Work out the finished part from the listing and answer in its coordinate system (mm). A direction names the side the tool comes from. Give positions to 0.01 mm unless a question says otherwise; leave off trailing zeros. Loops run counter-clockwise (first coordinate to the right, second up) from the corner with the lowest first, then second, coordinate; pieces in that order, holes last. Notation, with made-up numbers: M -28,22.5 L 13,22.5 A15 ccw 13,30.5 Z; hole C 54,-29 d2. An arc over 180 degrees is marked long. Use a Markdown table: item, result.
```python
from build123d import *

# Parameters (mm, degrees)
SKETCH1_R           = 25
BOSS_EXTRUDE1_DEPTH = 12
BOSS_EXTRUDE2_START = 12
SKETCH2_R           = 14
BOSS_EXTRUDE2_DEPTH = 7
CUT_EXTRUDE1_START  = 19
SKETCH3_R           = 11.15
CUT_EXTRUDE1_DEPTH  = 2.1
FILLET1_R           = 10
FILLET2_R           = 4
SKETCH4_R           = 11
BOSS_EXTRUDE3_DEPTH = 8
CUT_EXTRUDE2_START  = 16.9
SKETCH5_R           = 2.05
CUT_EXTRUDE2_DEPTH  = 9
SKETCH6_R           = 2.05
CUT_EXTRUDE3_DEPTH  = 9


with BuildPart() as part:
    # Sketch1 → Boss-Extrude1 (new body)
    with BuildSketch(Plane.XY):
        Circle(SKETCH1_R)
    extrude(amount=BOSS_EXTRUDE1_DEPTH)

    # Sketch2 → Boss-Extrude2 (add)
    with BuildSketch(Plane.XY.offset(BOSS_EXTRUDE2_START)):
        Circle(SKETCH2_R)
    extrude(amount=BOSS_EXTRUDE2_DEPTH)

    # Sketch3 → Cut-Extrude1 (cut)
    with BuildSketch(Plane.XY.offset(CUT_EXTRUDE1_START)):
        Circle(SKETCH3_R)
    extrude(amount=-CUT_EXTRUDE1_DEPTH, mode=Mode.SUBTRACT)

    # Fillet1
    # the kernel refuses this fillet: 10 mm, written as the material it adds along each edge
    with BuildSketch(Plane(origin=(0, 0, 12), x_dir=(1, 0, 0), z_dir=(0, -1, 0))) as fillet1_piece_1:
        with BuildLine():
            CenterArc((23.539392014, 10), FILLET1_R, 197.457603124, 72.542396876)
            Line((14, 7), (13.80921216, 6.94))
            ThreePointArc((13.80921216, 6.94), (13.8, 3.5), (13.8, 0))
            Line((13.8, 0), (14, -0.2))
            Line((14, -0.2), (23.539392014, -0.2))
            Line((23.539392014, -0.2), (23.539392014, 0))
        make_face()
    revolve(axis=Axis((0, 0, 12), (0, 0, 1)))

    # Fillet2
    fillet2_edges = [part.edges().sort_by_distance(p)[0] for p in [
        (-25, 0, 12),
    ]]
    fillet(fillet2_edges, radius=FILLET2_R)

    # Sketch4 → Boss-Extrude3 (add)
    with BuildSketch(Plane.XY):
        Circle(SKETCH4_R)
    extrude(amount=-BOSS_EXTRUDE3_DEPTH)

    # Sketch5 → Cut-Extrude2 (cut)
    with BuildSketch(Plane.XY.offset(CUT_EXTRUDE2_START)):
        with Locations((0, 8)):
            Circle(SKETCH5_R)
        with Locations((8, 0)):
            Circle(SKETCH5_R)
        with Locations((0, -8)):
            Circle(SKETCH5_R)
        with Locations((-8, 0)):
            Circle(SKETCH5_R)
    extrude(amount=-CUT_EXTRUDE2_DEPTH, mode=Mode.SUBTRACT)

    # Sketch6 → Cut-Extrude3 (cut)
    with BuildSketch(Plane.XY):
        with Locations((0, 18)):
            Circle(SKETCH6_R)
        with Locations((18, 0)):
            Circle(SKETCH6_R)
        with Locations((0, -18)):
            Circle(SKETCH6_R)
        with Locations((-18, 0)):
            Circle(SKETCH6_R)
    extrude(amount=CUT_EXTRUDE3_DEPTH, mode=Mode.SUBTRACT)


solid = part.part
```
(1) A cutting plane is placed at A-A (z = 7.25). Write down the section's boundary in (x, y), and give its area (3 significant figures).
Entries:
| item | result |
|---|---|
| outline | C 0,0 d50; hole C -18,0 d4.1; hole C 0,-18 d4.1; hole C 0,18 d4.1; hole C 18,0 d4.1 |
| area | 1,910 mm² |
(2) The mould has two halves that part along X. Classify faces 1 (the flat face through (0, -18, 9)), 2 (the flat face through (-1.1, -11.3, 19)), 3 (the cylindrical face through (23.846, 7.509, 4.058)): released by +X, released by -X, zero draft, split by the parting line, or undercut.
Entries:
| item | result |
|---|---|
| face 1 | undercut |
| face 2 | zero draft |
| face 3 | split by the parting line |
(3) A cutting plane is placed at B-B (z = -5.25). Write down the section's boundary in (x, y), and give its area (3 significant figures).
Entries:
| item | result |
|---|---|
| outline | C 0,0 d22 |
| area | 380 mm² |
(4) Which of the six approach directions +Z, -Z, +X, -X, +Y, -Y give full straight-line access (tool end or side, diameter ignored) to faces 4 (the flat face through (0, 0, -8)), 5 (the flat face through (8, 0, 7.9)), 6 (the cylindrical face through (-20.05, 0.09, 4.44))?
Entries:
| item | result |
|---|---|
| face 4 | -Z, +X, -X, +Y, -Y |
| face 5 | +Z |
| face 6 | -Z |
(5) Consider probe 1 along Y at (x, z) = (0, 4); probe 2 along Y at (x, z) = (8.5, 15.5); probe 3 along Y at (x, z) = (0, 14.75). Determine where each line is inside the solid, lowest interval first. Write a range as [from, to].
Entries:
| item | result |
|---|---|
| probe 1 | y = [-25, -20.05], [-15.95, 15.95], [20.05, 25] |
| probe 2 | y = [-13.48, -1.99], [1.99, 13.48] |
| probe 3 | y = [-16.65, -10.05], [-5.95, 5.95], [10.05, 16.65] |
(6) Given P1, Ø1, axis at x = -19.5, z = 1.5, coming from the +Y side; P2, Ø10, axis at x = -19.5, z = -2.5, coming from the -Y side; P3, Ø2.5, axis at x = 0, y = -18, coming from the +Z side, each flat-ended and moving along its own axis, determine where each tip first touches the part or whether it passes through.
Entries:
| item | result |
|---|---|
| P1 | stops at y = 16.25 |
| P2 | stops at y = -19.87 |
| P3 | stops at z = 14.66 |
